Read the model definition and answer for the solid it produces. Units are mm, in the model's axes. A direction names the side the tool comes from. Coordinates: 2 decimals unless noted, no trailing zeros. Write each loop counter-clockwise with the first axis right and the second up, starting at its lowest first coordinate (ties: lowest second). Pieces come first, ordered by that corner, then holes.
(1) Which of the six approach directions +Z, -Z, +X, -X, +Y, -Y give full straight-line access (tool end or side, diameter ignored) to faces 1 (the flat face through (0, 5, -1)), 2 (the flat face through (-1, 5, 6)), 3 (the flat face through (1, 5, -6))?
(2) Given pin 1 (0.6 mm diameter, centred on y = 5.5, z = 6.5, fed in from -X); pin 2 (6 mm diameter, centred on y = 8, z = 5, fed in from -X); pin 3 (1 mm diameter, centred on y = 7, z = 6.5, fed in from +X), each flat-ended and moving along its own axis, determine where each tip first touches the part or whether it passes through.
(3) The part is cut by section A-A, the plane x = 0. Determine the outline of the cut face in (y, z), and give its area (3 significant figures).
(4) The part is cut by section B-B, the plane y = 5.5. Determine the outline of the cut face in (x, z).
(5) Determine the mould class of faces 4 (the cylindrical face through (-7.5, 4.93, -0.15)), 5 (the flat face through (1, 5, 6)), 6 (the flat face through (0, 10, 2)) for opening direction X: pulls with the +X half, pulls with the -X half, needs draft (parallel to the pull), parting line crosses it, or undercut.
(6) The part is cut by section C-C, the plane z = -0.5. Determine the outline of the cut face in (x, y).
(7) Straight lines are drawn through the part: line 1 along Z through (x, y) = (0, 2.5); line 2 along X through (y, z) = (3.25, 0); line 3 along Z through (x, y) = (-1.25, 1.5). For each, find the intervals that lie inside material, in ascending order.
(8) The part is cut by section D-D, the plane x = -4.75. Determine the outline of the cut face in (y, z), and give its area (3 significant figures).
```python
from build123d import *

# Parameters (mm, degrees)
EXTRUDE_1_DEPTH = 10


with BuildPart() as part:
    # Эскиз1 → Бобышка-Вытянуть1 (new body)
    # profile 1 of 2: a face of its own
    with BuildSketch(Plane(origin=(0, 0, 0), x_dir=(1, 0, 0), z_dir=(0, 1, 0))):
        with BuildLine():
            Line((-1, 5.5), (-1, 7.433034374))
            ThreePointArc((-1, 7.433034374), (-7.5, 0), (-1, -7.433034374))
            Line((-1, -7.433034374), (-1, -5.5))
            Line((-1, -5.5), (1, -5.5))
            Line((1, -5.5), (1, -7.433034374))
            ThreePointArc((1, -7.433034374), (5.645794895, -4.937104415), (7.5, 0))
            ThreePointArc((7.5, 0), (5.645794895, 4.937104415), (1, 7.433034374))
            Line((1, 7.433034374), (1, 5.5))
            Line((1, 5.5), (-1, 5.5))
        make_face()
        with BuildLine():
            ThreePointArc((1.5, 0), (-0.535233135, -1.401258538), (-1.118033989, 1))
            ThreePointArc((-1.118033989, 1), (0, 1.5), (1.118033989, 1))
            ThreePointArc((1.118033989, 1), (1.401258538, 0.535233135), (1.5, 0))
        make_face(mode=Mode.SUBTRACT)
    # profile 2 of 2: a face of its own
    with BuildSketch(Plane(origin=(0, 0, 0), x_dir=(1, 0, 0), z_dir=(0, 1, 0))):
        with BuildLine():
            ThreePointArc((1.118033989, 1), (0, 1.5), (-1.118033989, 1))
            Line((-1.118033989, 1), (1.118033989, 1))
        make_face()
    extrude(amount=EXTRUDE_1_DEPTH)


solid = part.part
```
Computed:
1. face 1: +Y, -Y
1. face 2: +Z, +Y, -Y
1. face 3: -Z, +Y, -Y
2. pin 1: stops at x = -4.22
2. pin 2: stops at x = -7.23
2. pin 3: stops at x = 4.5
3. outline: (0, -5.5) - (10, -5.5) - (10, -1) - (0, -1) - close; (0, 1.5) - (10, 1.5) - (10, 5.5) - (0, 5.5) - close
3. area: 85.0 mm2
4. outline: (-1, -7.43) - (-1, -5.5) - (1, -5.5) - (1, -7.43) arc R7.5 ccw to (1, 7.43) - (1, 5.5) - (-1, 5.5) - (-1, 7.43) arc R7.5 ccw to start; hole (-1.12, -1) - (1.12, -1) arc R1.5 ccw (long way) to start
5. face 4: pulls with the -X half
5. face 5: undercut
5. face 6: needs draft
6. outline: (-7.48, 0) - (-1.41, 0) - (-1.41, 10) - (-7.48, 10) - close; (1.41, 0) - (7.48, 0) - (7.48, 10) - (1.41, 10) - close
7. line 1: z = -5.5 to -1, 1.5 to 5.5
7. line 2: x = -7.5 to -1.5, 1.5 to 7.5
7. line 3: z = -7.4 to -0.83, 0.83 to 7.4
8. outline: (0, -5.8) - (10, -5.8) - (10, 5.8) - (0, 5.8) - close
8. area: 116 mm2
